For this review, take the finished solid that the model builds, in its own axes (mm). Face numbers are marked on the shaded views. A direction names the side the tool comes from. Coordinates: 2 decimals unless noted, no trailing zeros. Loops run counter-clockwise (first coordinate to the right, second up) from the corner with the lowest first, then second, coordinate; pieces in that order, holes last. Notation, with made-up numbers: (29.5, 26) - (36.5, 26) arc R20 cw to (36.5, 43) - close; hole circle Ø11 at (21, 14.25). An arc over 180 degrees is marked (long way). Use one line per item in the form item = value. Start each with the question number.
1. Add section D-D on y = -4. Give the boundary of the cut face in (x, z).
2. Add section B-B on z = 0. Give the boundary of the cut face in (x, y), and give its area (3 significant figures).
3. Draft analysis for pull direction X (two halves, no side actions). For the marked faces 1, 2 and 3, state which applies: +X half, -X half, draft (parallel to the pull), parting line (faces both ways), or undercut.
4. Add section C-C on x = -4.5. Give the boundary of the cut face in (y, z), and give its area (3 significant figures).
5. For pin 1 Ø6 at (x, y) = (3.5, -19) entering from -Z; pin 2 Ø1.5 at (x, y) = (0, -8.82) entering from -Z; pin 3 Ø2 at (x, y) = (5, -15) entering from -Z, all flat-tipped, find the tip position at first contact; note any pin that passes through.
6. Machinability: for the marked faces 4 and 5, which of the approach directions +Z, -Z, +X, -X, +Y, -Y give a long, thin tool a straight path to every point of the face, cutting with its end or side? Answer none if there is none.
7. Add section A-A on x = 0. Give the boundary of the cut face in (y, z), and give its area (3 significant figures).
8. To check wall thickness, follow probe 1 along Y at (x, z) = (-1.25, 6); probe 2 along Y at (x, z) = (0, -6.95); probe 3 along Y at (x, z) = (-1, -6). State the ranges of each line that lie inside material, in increasing order.
```python
from build123d import *

# Parameters (mm, degrees)
CUT_EXTRUDE1_REACH = 31.736
SKETCH2_R          = 4
SKETCH3_R          = 1.25
CUT_EXTRUDE2_DEPTH = 10
CIRPATTERN1_COUNT  = 2
CIRPATTERN1_ANGLE  = 90


with BuildPart() as part:
    # Sketch1 → Revolve1 (revolve)
    with BuildSketch(Plane.XY):
        Polygon((0, 5), (-8, 5), (-8, 3.5), (-6, 3.5), (-6, -5.5), (-8, -5.5), (-8, -12), (-6, -12), (-6, -21), (-8, -21), (-8, -22.5), (0, -22.5), align=None)
    revolve(axis=Axis((0, 291.267844828, 0), (0, -1, 0)))

    # Sketch2 → Cut-Extrude1 (cut, up to next)
    with BuildSketch(Plane(origin=(0, 5, 0), x_dir=(1, 0, 0), z_dir=(0, 1, 0)), mode=Mode.PRIVATE) as cut_extrude1_sk1:
        with Locations(Location((0, 0, 0), (0, 0, 180))):
            Circle(SKETCH2_R)
    cut_extrude1_tool1 = extrude(cut_extrude1_sk1.sketch, amount=-CUT_EXTRUDE1_REACH, mode=Mode.PRIVATE) & part.part
    add(cut_extrude1_tool1.solids().sort_by_distance((0, 5, 0))[0], mode=Mode.SUBTRACT)

    # Sketch3 → Cut-Extrude2 (cut)
    with BuildSketch(Plane.XY):
        with Locations((0, -8.820149855)):
            Circle(SKETCH3_R)
    cut_extrude2 = extrude(amount=-CUT_EXTRUDE2_DEPTH, mode=Mode.SUBTRACT)

    # CirPattern1: Cut-Extrude2 ×2 about axis
    cirpattern1_axis = Axis((0, -22.5, 0), (0, 1, 0))
    for i in range(1, CIRPATTERN1_COUNT):
        add(cut_extrude2.rotate(cirpattern1_axis, i * CIRPATTERN1_ANGLE / (CIRPATTERN1_COUNT - 1)), mode=Mode.SUBTRACT)


solid = part.part
```
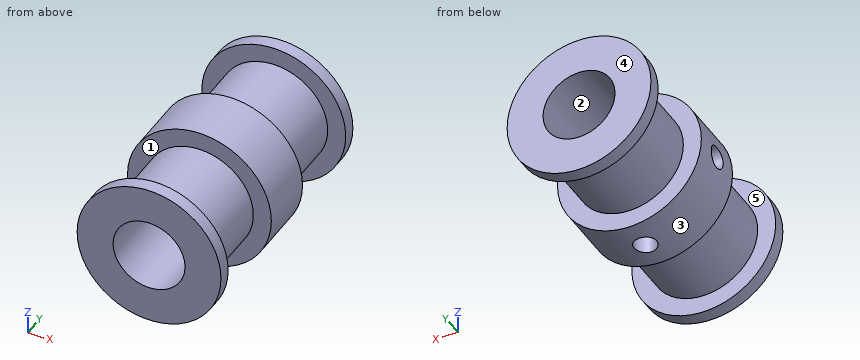
Conclusion:
q1.outline = circle Ø12 at (0, 0); hole circle Ø8 at (0, 0)
q2.outline = (-8, -22.5) - (-4, -22.5) - (-4, -10.07) - (-8, -10.07) - (-8, -12) - (-6, -12) - (-6, -21) - (-8, -21) - close; (-8, -7.57) - (-4, -7.57) - (-4, 5) - (-8, 5) - (-8, 3.5) - (-6, 3.5) - (-6, -5.5) - (-8, -5.5) - close; (4, -22.5) - (8, -22.5) - (8, -21) - (6, -21) - (6, -12) - (8, -12) - (8, -5.5) - (6, -5.5) - (6, 3.5) - (8, 3.5) - (8, 5) - (4, 5) - close
q2.area = 138 mm^2
q3.face_1 = draft
q3.face_2 = undercut
q3.face_3 = parting line
q4.outline = (-22.5, -6.61) - (-21, -6.61) - (-21, -3.97) - (-12, -3.97) - (-12, -6.61) - (-5.5, -6.61) - (-5.5, -3.97) - (3.5, -3.97) - (3.5, -6.61) - (5, -6.61) - (5, 6.61) - (3.5, 6.61) - (3.5, 3.97) - (-5.5, 3.97) - (-5.5, 6.61) - (-12, 6.61) - (-12, 3.97) - (-21, 3.97) - (-21, 6.61) - (-22.5, 6.61) - close; hole circle Ø2.5 at (-8.82, 0)
q4.area = 264 mm^2
q5.pin_1 = -7.9
q5.pin_2 = 3.93
q5.pin_3 = -4.47
q6.face_4 = +Z, -Z, +X, -X, +Y
q6.face_5 = none
q7.outline = (-22.5, -8) - (-21, -8) - (-21, -6) - (-12, -6) - (-12, -8) - (-10.07, -8) - (-10.07, -4) - (-22.5, -4) - close; (-22.5, 4) - (5, 4) - (5, 8) - (3.5, 8) - (3.5, 6) - (-5.5, 6) - (-5.5, 8) - (-12, 8) - (-12, 6) - (-21, 6) - (-21, 8) - (-22.5, 8) - close; (-7.57, -8) - (-5.5, -8) - (-5.5, -6) - (3.5, -6) - (3.5, -8) - (5, -8) - (5, -4) - (-7.57, -4) - close
q7.area = 138 mm^2
q8.probe_1 = -22.5 to -21, -12 to -5.5, 3.5 to 5
q8.probe_2 = -22.5 to -21, -12 to -10.07, -7.57 to -5.5, 3.5 to 5
q8.probe_3 = -22.5 to -21, -12 to -9.57, -8.07 to -5.5, 3.5 to 5
